Read the model definition and answer for the solid it produces. Units are mm, in the model's axes. Face numbers are marked on the shaded views. A direction names the side the tool comes from. Round coordinates to 2 decimals unless told otherwise and drop trailing zeros. Order: outer loops, then holes, each group sorted by start corner. A loop starts at its lowest first (then second) coordinate and runs counter-clockwise, first axis right, second up. Notation, with made-up numbers: (-17.75, -17) -> (2.25, -17) arc R16 ccw to (2.25, -5) -> close; hole circle Ø4 at (10, -10). An arc over 180 degrees is marked (long way). One line per item, written item: value. Start each with the question number.
1. For the marked faces 5 and 6, determine the directions among +Z, -Z, +X, -X, +Y, -Y from which every point of the face is accessible in a straight line to the end or side of a thin tool.
2. Consider line 1 (Y direction, x = 15, z = -7); line 2 (Y direction, x = 15, z = -6); line 3 (X direction, y = -15.5, z = -17). Determine where each line is inside the solid, lowest interval first.
3. The mould has two halves that part along X. Classify the marked faces 1, 2, 3 and 4: released by +X, released by -X, zero draft, split by the parting line, or undercut.
4. Section B-B (z = -6) is taken. Give the vertices of the cut face in (x, y), then the cut area to 3 significant figures.
5. Section A-A (y = 15) is taken. Give the vertices of the cut face in (x, z), then the cut area to 3 significant figures.
6. Flat-ended cylindrical pins translate along their axes: pin 1 Ø10 at (x, z) = (13, -13) entering from +Y; pin 2 Ø4 at (x, y) = (27.5, 15.5) entering from -Z; pin 3 Ø2 at (y, z) = (-24.5, -10) entering from -X; pin 4 Ø3 at (x, y) = (22.5, -29) entering from +Z. Find the tip coordinate at first contact, or state that the pin passes through.
7. Section C-C (x = 26.5) is taken. Give the vertices of the cut face in (y, z), then the cut area to 4 significant figures.
8. Section D-D (z = -26) is taken. Give the vertices of the cut face in (x, y), then the cut area to 3 significant figures.
from build123d import *

# Parameters (mm, degrees)
SKETCH_1_W      = 30
SKETCH_1_H      = 30
EXTRUDE_1_DEPTH = 10
EXTRUDE_2_DEPTH = 5
EXTRUDE_3_DEPTH = 5
SKETCH_6_W      = 5
SKETCH_6_H      = 8
EXTRUDE_4_DEPTH = 1.5


# Read off the part's stored shape, not the designer's step: 高级异型孔1, 高级异型孔2
with BuildPart() as part:
    # 草图1 → 凸台-拉伸1 (new body)
    with BuildSketch(Plane.XY):
        with Locations((15, 15)):
            Rectangle(SKETCH_1_W, SKETCH_1_H)
    extrude(amount=EXTRUDE_1_DEPTH)

    # 草图2 → 凸台-拉伸2 (add)
    with BuildSketch(Plane.XZ):
        Polygon((0, 10), (30, 10), (30, 0), (20, -30), (10, -30), (0, 0), align=None)
    extrude(amount=EXTRUDE_2_DEPTH)

    # 草图3 → 凸台-拉伸3 (add, symmetric)
    with BuildSketch(Plane(origin=(15, 0, 0), x_dir=(0, 0, -1), z_dir=(1, 0, 0))):
        with BuildLine():
            Line((0, -48), (0, -58))
            Line((0, -58), (18, -58))
            Line((18, -58), (30, -5))
            Line((30, -5), (-10, -5))
            Line((-10, -5), (0, -22))
            Line((0, -22), (0, -32))
            ThreePointArc((0, -32), (8, -40), (0, -48))
        make_face()
    extrude(amount=EXTRUDE_3_DEPTH, both=True)

    # 草图6 → 凸台-拉伸4 (add, symmetric)
    with BuildSketch(Plane(origin=(0, 0, 0), x_dir=(-1, 0, 0), z_dir=(0, 0, -1))):
        with Locations((-27.5, 15)):
            Rectangle(SKETCH_6_W, SKETCH_6_H)
        with Locations((-2.5, 15)):
            Rectangle(SKETCH_6_W, SKETCH_6_H)
    extrude(amount=EXTRUDE_4_DEPTH, both=True)

    # 高级异型孔1 outline → 高级异型孔1 (revolve, cut)
    with BuildSketch(Plane(origin=(15, 15, 0), x_dir=(1, 0, 0), z_dir=(0, -1, 0))):
        Polygon((3.15, 10), (0, 10), (0, 0), (1.7, 0), (1.7, 8.55), align=None)
    revolve(axis=Axis((15, 15, 0), (0, 0, 1)), mode=Mode.SUBTRACT)

    # 高级异型孔2 outline → 高级异型孔2 (revolve, cut)
    with BuildSketch(Plane(origin=(15, -53, 0), x_dir=(1, 0, 0), z_dir=(0, -1, 0))):
        Polygon((0, -10.991420021), (1.65, -10), (1.65, 0), (0, 0), align=None)
    revolve(axis=Axis((15, -53, 0), (0, 0, 1)), mode=Mode.SUBTRACT)

    # Other 2 2 outline → Other 2 2 (revolve, cut)
    with BuildSketch(Plane(origin=(15, -27, 0), x_dir=(1, 0, 0), z_dir=(0, -1, 0))):
        Polygon((0, -10.991420021), (1.65, -10), (1.65, 0), (0, 0), align=None)
    revolve(axis=Axis((15, -27, 0), (0, 0, 1)), mode=Mode.SUBTRACT)


solid = part.part
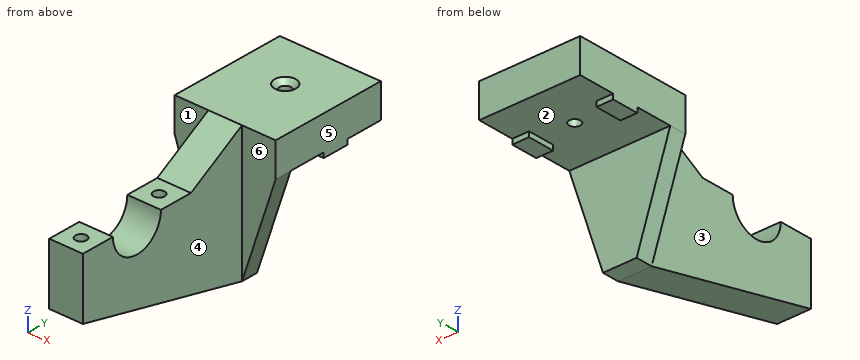
Answer:
1. face 5: +Z, -Z, +X, +Y, -Y
1. face 6: +Z, -Z, +X, -Y
2. line 1: -58 to -54.65, -51.35 to -43.87, -36.13 to -28.65, -25.35 to 0
2. line 2: -58 to -54.65, -51.35 to -45.29, -34.71 to -28.65, -25.35 to 0
2. line 3: 10 to 20
3. face 1: zero draft
3. face 2: undercut
3. face 3: released by -X
3. face 4: released by +X
4. outline: (2, -5) -> (10, -5) -> (10, -34.71) -> (20, -34.71) -> (20, -5) -> (28, -5) -> (28, 0) -> (2, 0) -> close; (10, -58) -> (20, -58) -> (20, -45.29) -> (10, -45.29) -> close; hole circle Ø3.3 at (15, -53); hole circle Ø3.3 at (15, -27)
4. area: 537 mm^2
5. outline: (0, -1.5) -> (5, -1.5) -> (5, 0) -> (13.3, 0) -> (13.3, 8.55) -> (11.85, 10) -> (0, 10) -> close; (16.7, 0) -> (25, 0) -> (25, -1.5) -> (30, -1.5) -> (30, 10) -> (18.15, 10) -> (16.7, 8.55) -> close
5. area: 279 mm^2
6. pin 1: y = 0
6. pin 2: z = -1.5
6. pin 3: x = 10
6. pin 4: through
7. outline: (-5, -10.5) -> (0, -10.5) -> (0, 0) -> (11, 0) -> (11, -1.5) -> (19, -1.5) -> (19, 0) -> (30, 0) -> (30, 10) -> (-5, 10) -> close
7. area: 414.5 mm^2
8. outline: (8.67, -5) -> (10, -5) -> (10, -22.67) -> (20, -22.67) -> (20, -5) -> (21.33, -5) -> (21.33, 0) -> (8.67, 0) -> close
8. area: 240 mm^2
